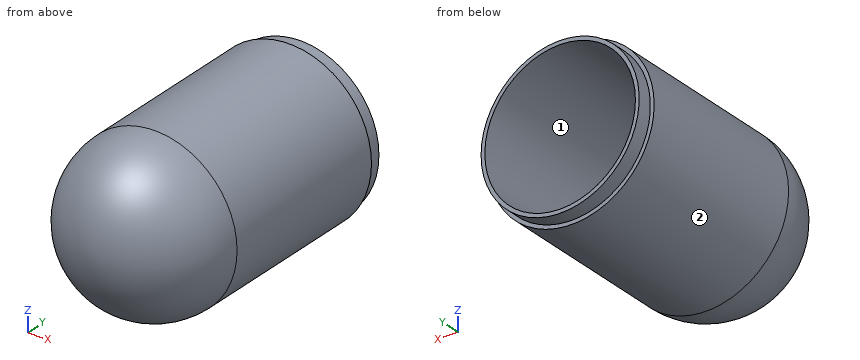
from build123d import *

# Parameters (mm, degrees)
SKETCH3_R           = 69.85
CUT_EXTRUDE1_DEPTH  = 12.7
SKETCH4_R           = 66.675
SKETCH4_R_2         = 63.5
BOSS_EXTRUDE2_DEPTH = 12.7
SKETCH5_R           = 68.2625
SKETCH5_R_2         = 66.675
BOSS_EXTRUDE3_DEPTH = 9.525
SKETCH7_R           = 68.2625
SKETCH7_R_2         = 66.675
CUT_EXTRUDE2_DEPTH  = 1.5875
SKETCH12_R          = 68.2625
SKETCH12_R_2        = 66.675
CUT_EXTRUDE3_DEPTH  = 7.9375


with BuildPart() as part:
    # Sketch1 → Revolve1 (revolve)
    with BuildSketch(Plane.XY):
        with BuildLine():
            Line((63.5, 0), (63.5, 152.4))
            Line((63.5, 152.4), (66.675, 152.4))
            Line((66.675, 152.4), (66.675, 165.1))
            Line((66.675, 165.1), (69.85, 165.1))
            Line((69.85, 165.1), (69.85, 152.4))
            Line((69.85, 152.4), (69.85, 0))
            ThreePointArc((69.85, 0), (49.391408666, -49.391408666), (0, -69.85))
            Line((0, -69.85), (0, -63.5))
            ThreePointArc((0, -63.5), (44.901280605, -44.901280605), (63.5, 0))
        make_face()
    revolve(axis=Axis((0, -63.5, 0), (0, -1, 0)))

    # Sketch3 → Cut-Extrude1 (cut)
    with BuildSketch(Plane(origin=(0, 165.1, 0), x_dir=(1, 0, 0), z_dir=(0, 1, 0))):
        Circle(SKETCH3_R)
    extrude(amount=-CUT_EXTRUDE1_DEPTH, mode=Mode.SUBTRACT)

    # Sketch4 → Boss-Extrude2 (add)
    with BuildSketch(Plane(origin=(0, 152.4, 0), x_dir=(1, 0, 0), z_dir=(0, 1, 0))):
        Circle(SKETCH4_R)
        Circle(SKETCH4_R_2, mode=Mode.SUBTRACT)
    extrude(amount=BOSS_EXTRUDE2_DEPTH)

    # Sketch5 → Boss-Extrude3 (add)
    with BuildSketch(Plane(origin=(0, 165.1, 0), x_dir=(1, 0, 0), z_dir=(0, 1, 0))):
        Circle(SKETCH5_R)
        Circle(SKETCH5_R_2, mode=Mode.SUBTRACT)
    extrude(amount=-BOSS_EXTRUDE3_DEPTH)

    # Sketch7 → Cut-Extrude2 (cut)
    with BuildSketch(Plane(origin=(0, 165.1, 0), x_dir=(1, 0, 0), z_dir=(0, 1, 0))):
        Circle(SKETCH7_R)
        Circle(SKETCH7_R_2, mode=Mode.SUBTRACT)
    extrude(amount=-CUT_EXTRUDE2_DEPTH, mode=Mode.SUBTRACT)

    # Sketch12 → Cut-Extrude3 (cut)
    with BuildSketch(Plane(origin=(0, 163.5125, 0), x_dir=(1, 0, 0), z_dir=(0, 1, 0))):
        Circle(SKETCH12_R)
        Circle(SKETCH12_R_2, mode=Mode.SUBTRACT)
    extrude(amount=-CUT_EXTRUDE3_DEPTH, mode=Mode.SUBTRACT)


solid = part.part
Model file for the job. Use its own axes, mm. Face numbers are marked on the shaded views. Give positions to 0.01 mm unless a question says otherwise; leave off trailing zeros. Order: outer loops, then holes, each group sorted by start corner. A loop starts at its lowest first (then second) coordinate and runs counter-clockwise, first axis right, second up. Notation, with made-up numbers: (50.5, -4) - (87.5, -4) arc R23 cw to (87.5, 31) - close; hole circle Ø9 at (20.5, 7). An arc over 180 degrees is marked (long way). One line per item, written item: value.
Item 1: Pin check, flat tips, straight feed: pin 1 Ø1 at (x, y) = (3.5, 111) entering from -Z; pin 2 Ø4 at (x, y) = (-28.5, -45) entering from +Z; pin 3 Ø3 at (x, z) = (9, -46.5) entering from +Y; pin 4 Ø12 at (y, z) = (23, -0.5) entering from -X. Stop position of each tip, or through.
Response values:
pin 1: z = -69.79
pin 2: z = 47.44
pin 3: y = -40.55
pin 4: x = -69.85
Item 2: Wall check: line 1 (X direction, y = 93, z = -0.5); line 2 (Y direction, x = 1.5, z = -2). Give the ranges that are in metal, low to high.
Response values:
line 1: -69.85 to -63.5, 63.5 to 69.85
line 2: -69.81 to -63.45
Item 3: Slice it at C-C (y = 29.5). List the corners of the cut face in (x, z), then the cut area to 3 significant figures.
Response values:
outline: circle Ø139.7 at (0, 0); hole circle Ø127 at (0, 0)
area: 2,660 mm2
Item 4: Two-plate mould, pull along X, no slides. Class the marked faces 1 and 2: released by +X, released by -X, zero draft, split by the parting line, or undercut.
Response values:
face 1: undercut
face 2: split by the parting line
Item 5: Slice it at A-A (x = 0). List the corners of the cut face in (y, z) (3 decimals), then the cut area to 3 significant figures.
Response values:
outline: (0, -69.85) - (152.4, -69.85) - (152.4, -66.675) - (165.1, -66.675) - (165.1, -63.5) - (0, -63.5) arc R63.5 cw to (0, 63.5) - (165.1, 63.5) - (165.1, 66.675) - (152.4, 66.675) - (152.4, 69.85) - (0, 69.85) arc R69.85 ccw to start
area: 3,350 mm2
Item 6: Slice it at B-B (z = 0). List the corners of the cut face in (x, y) (3 decimals).
Response values:
outline: (-69.85, 0) arc R69.85 ccw to (69.85, 0) - (69.85, 152.4) - (66.675, 152.4) - (66.675, 165.1) - (63.5, 165.1) - (63.5, 0) arc R63.5 cw to (-63.5, 0) - (-63.5, 165.1) - (-66.675, 165.1) - (-66.675, 152.4) - (-69.85, 152.4) - close
Item 7: Slice it at D-D (z = 36.5). List the corners of the cut face in (x, y).
Response values:
outline: (-59.55, 0) arc R59.55 ccw to (59.55, 0) - (59.55, 152.4) - (55.8, 152.4) - (55.8, 165.1) - (51.96, 165.1) - (51.96, 0) arc R51.96 cw to (-51.96, 0) - (-51.96, 165.1) - (-55.8, 165.1) - (-55.8, 152.4) - (-59.55, 152.4) - close
